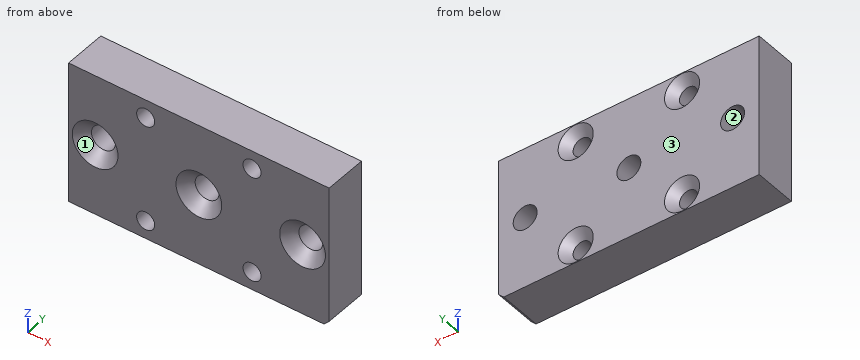
from build123d import *

# Parameters (mm, degrees)
SKETCH_1_W                   = 49
SKETCH_1_H                   = 26.8
EXTRUDE_1_DEPTH              = 8
HOLE_WIZARD_M3_1_D           = 3.4
HOLE_WIZARD_M3_1_CSINK_D     = 6.6
HOLE_WIZARD_M3_1_CSINK_ANGLE = 90
HOLE_WIZARD_M4_1_D           = 4.5
HOLE_WIZARD_M4_1_CSINK_D     = 8.6
HOLE_WIZARD_M4_1_CSINK_ANGLE = 90
CHAMFER_1_SIZE               = 1


with BuildPart() as part:
    # 草图1 → 凸台-拉伸1 (new body)
    with BuildSketch(Plane(origin=(0, 0, 0), x_dir=(1, 0, 0), z_dir=(0, 1, 0))):
        Rectangle(SKETCH_1_W, SKETCH_1_H)
    extrude(amount=EXTRUDE_1_DEPTH)

    # M3 十字槽沉头木螺钉的锥形沉头孔1 (through all)
    with Locations(Plane(origin=(0, 8, 0), x_dir=(1, 0, 0), z_dir=(0, 1, 0))):
        with Locations((-10, -10), (10, -10), (10, 10), (-10, 10)):
            CounterSinkHole(HOLE_WIZARD_M3_1_D / 2, HOLE_WIZARD_M3_1_CSINK_D / 2, counter_sink_angle=HOLE_WIZARD_M3_1_CSINK_ANGLE)

    # M4 十字槽沉头木螺钉的锥形沉头孔1 (through all)
    with Locations(Plane(origin=(0, 0, 0), x_dir=(-1, 0, 0), z_dir=(0, -1, 0))):
        with Locations((19.5, 0), (0, 0), (-19.5, 0)):
            CounterSinkHole(HOLE_WIZARD_M4_1_D / 2, HOLE_WIZARD_M4_1_CSINK_D / 2, counter_sink_angle=HOLE_WIZARD_M4_1_CSINK_ANGLE)

    # 倒角1
    chamfer_1_edges = [part.edges().sort_by_distance(p)[0] for p in [
        (24.5, 4, -13.4),
    ]]
    chamfer(chamfer_1_edges, length=CHAMFER_1_SIZE)


solid = part.part
Read the model definition and answer for the solid it produces. Units are mm, in the model's axes. Face numbers are marked on the shaded views. Round coordinates to 2 decimals unless told otherwise and drop trailing zeros. Write each loop counter-clockwise with the first axis right and the second up, starting at its lowest first coordinate (ties: lowest second). Pieces come first, ordered by that corner, then holes. Notation, with made-up numbers: (14, 70.25) - (62, 70.25) arc R21 ccw to (62, 82.25) - close; hole circle Ø10 at (62.5, 20). An arc over 180 degrees is marked (long way). Use a Markdown table: item, result.
(1) The part is cut by section B-B (x = -10). Write down the section's boundary in (y, z), then the cut area to 3 significant figures.
Reported:
| item | result |
|---|---|
| outline | (0, -13.4) - (8, -13.4) - (8, -13.3) - (6.4, -11.7) - (0, -11.7) - close; (0, -8.3) - (6.4, -8.3) - (8, -6.7) - (8, 6.7) - (6.4, 8.3) - (0, 8.3) - close; (0, 11.7) - (6.4, 11.7) - (8, 13.3) - (8, 13.4) - (0, 13.4) - close |
| area | 155 mm2 |
(2) The part is cut by section D-D (z = -10). Write down the section's boundary in (x, y), then the cut area to 3 significant figures.
Reported:
| item | result |
|---|---|
| outline | (-24.5, 0) - (-11.7, 0) - (-11.7, 6.4) - (-13.3, 8) - (-24.5, 8) - close; (-8.3, 0) - (8.3, 0) - (8.3, 6.4) - (6.7, 8) - (-6.7, 8) - (-8.3, 6.4) - close; (11.7, 0) - (24.5, 0) - (24.5, 8) - (13.3, 8) - (11.7, 6.4) - close |
| area | 332 mm2 |
(3) Straight lines are drawn through the part: line 1 along Z through (x, y) = (10, 2.75); line 2 along X through (y, z) = (1.75, -10); line 3 along Z through (x, y) = (19.5, 4.8). For each, find the intervals that lie inside material, in ascending order. Write a range as [from, to].
Reported:
| item | result |
|---|---|
| line 1 | [-13.4, -11.7], [-8.3, 8.3], [11.7, 13.4] |
| line 2 | [-24.5, -11.7], [-8.3, 8.3], [11.7, 24.5] |
| line 3 | [-13.4, -2.25], [2.25, 13.4] |
(4) The part is cut by section C-C (x = 0). Write down the section's boundary in (y, z), then the cut area to 3 significant figures.
Reported:
| item | result |
|---|---|
| outline | (0, -13.4) - (8, -13.4) - (8, -2.25) - (2.05, -2.25) - (0, -4.3) - close; (0, 4.3) - (2.05, 2.25) - (8, 2.25) - (8, 13.4) - (0, 13.4) - close |
| area | 174 mm2 |
(5) The part is cut by section A-A (z = 0). Write down the section's boundary in (x, y), then the cut area to 3 significant figures.
Reported:
| item | result |
|---|---|
| outline | (-24.5, 0) - (-23.8, 0) - (-21.75, 2.05) - (-21.75, 8) - (-24.5, 8) - close; (-17.25, 2.05) - (-15.2, 0) - (-4.3, 0) - (-2.25, 2.05) - (-2.25, 8) - (-17.25, 8) - close; (2.25, 2.05) - (4.3, 0) - (15.2, 0) - (17.25, 2.05) - (17.25, 8) - (2.25, 8) - close; (21.75, 2.05) - (23.8, 0) - (24.5, 0) - (24.5, 8) - (21.75, 8) - close |
| area | 271 mm2 |
(6) Each of these flat-tipped pins is pushed along its axis until it touches: pin 1 Ø2.5 at (x, z) = (-10, -10) entering from -Y; pin 2 Ø1 at (x, z) = (-0.5, -7.5) entering from -Y. Where does it stop, or does it pass through?
Reported:
| item | result |
|---|---|
| pin 1 | through |
| pin 2 | y = 0 |
(7) The mould has two halves that part along Y. Classify the marked faces 1, 2 and 3: released by +Y, released by -Y, zero draft, split by the parting line, or undercut.
Reported:
| item | result |
|---|---|
| face 1 | released by -Y |
| face 2 | zero draft |
| face 3 | released by +Y |
